Solid Edge part; units mm, degrees
sketch "Sketch1" plane through (0, 0, 0) normal (0, -1, 0) x (1, 0, 0)
  line L0 (4, 2.3094) -> (0, 4.6188)
  line L1 (0, 4.6188) -> (-4, 2.3094)
  line L2 (-4, 2.3094) -> (-4, -2.3094)
  line L3 (-4, -2.3094) -> (0, -4.6188)
  line L4 (0, -4.6188) -> (4, -2.3094)
  line L5 (4, -2.3094) -> (4, 2.3094)
extrude "Protrusion1" add sketch "Sketch1" along normal mid plane 2.7
sketch "Sketch2" plane through (0, 0, 0) normal (1, 0, 0) x (0, 1, 0)
  line L0 (-1.35, 3.45) -> (-1.0368, 4.6188)
revolve "RevolvedCutout1" cut sketch "Sketch2" angle 360 about axis through (0, 0, 0) along (0, -1, 0) material side at (0, -1.2417, 4.0473)
mirror "Mirror1" about plane through (0, 0, 0) normal (0, -1, 0) of "RevolvedCutout1"
hole "孔_7" at (0, -1.35, 0) direction (0, 1, 0) diameter 4.134 end up to next start chamfer 0.5 start chamfer angle 60 end chamfer 0.5 end chamfer angle 60
Check sheet for the modelled part. Datum: model origin and axes. Units: mm. Coordinates: 2 decimals unless noted, no trailing zeros. Loops run counter-clockwise (first coordinate to the right, second up) from the corner with the lowest first, then second, coordinate; pieces in that order, holes last. Notation, with made-up numbers: (2, 6) -> (45, 6) arc R24 cw to (45, 45) -> close; hole circle Ø10 at (54.25, 68). An arc over 180 degrees is marked (long way). Write item = value, one per line. Start each with the question number.
1. Draft check along Z on faces 1 (the cylindrical face through (-1.26, -0.01, 1.64)), 2 (the flat face through (1.97, 0.02, -3.48)), 3 (the flat face through (3, -1.35, 0)). Enter one of: released by +Z, released by -Z, zero draft, split by the parting line, or undercut.
2. Depth check by flat-ended pin: P1, Ø3.5, axis at x = 0, z = 0, coming from the -Y side. Enter the tip coordinate at first touch or a pass-through.
3. Material ranges on line 1 (X direction, y = 0.25, z = 0); line 2 (X direction, y = -0.5, z = -1.5); line 3 (X direction, y = -0.15, z = -3.25), recorded low to high.
4. Section check B-B on y = 0.8. Record the cut outline in (x, z).
5. Section check A-A on z = 0. Record the cut outline in (x, y), then the cut area to 3 significant figures.
Responses:
q1.face_1 = undercut
q1.face_2 = released by -Z
q1.face_3 = zero draft
q2.P1 = through
q3.line_1 = -4 to -2.07, 2.07 to 4
q3.line_2 = -4 to -1.42, 1.42 to 4
q3.line_3 = -2.37 to 2.37
q4.outline = (-4, -2.31) -> (0, -4.62) -> (4, -2.31) -> (4, 2.31) -> (0, 4.62) -> (-4, 2.31) -> close; hole circle Ø4.13 at (0, 0)
q5.outline = (-4, -1.2) -> (-3.45, -1.35) -> (-2.57, -1.35) -> (-2.07, -1.06) -> (-2.07, 1.06) -> (-2.57, 1.35) -> (-3.45, 1.35) -> (-4, 1.2) -> close; (2.07, -1.06) -> (2.57, -1.35) -> (3.45, -1.35) -> (4, -1.2) -> (4, 1.2) -> (3.45, 1.35) -> (2.57, 1.35) -> (2.07, 1.06) -> close
q5.area = 9.99 mm2
